from build123d import *

# Parameters (mm, degrees)
CROQUIS2_R               = 2.5
SALIENTE_EXTRUIR1_DEPTH  = 8
CROQUIS3_R               = 3.5
CORTAR_EXTRUIR1_DEPTH    = 1
CORTAR_EXTRUIR2_START    = -1
CROQUIS4_R               = 3.5
CORTAR_EXTRUIR2_DEPTH    = 1
BOSS_EXTRUDE1_DEPTH      = 10
BOSS_EXTRUDE1_DEPTH_BACK = 18
CUT_EXTRUDE1_DEPTH       = 10
CUT_EXTRUDE2_DEPTH       = 46
CUT_EXTRUDE2_DEPTH_BACK  = 31


with BuildPart() as part:
    # Croquis2 → Saliente-Extruir1 (new body)
    with BuildSketch(Plane(origin=(0, 0, 0), x_dir=(1, 0, 0), z_dir=(0, 1, 0))):
        with BuildLine():
            Line((-6.5, 70), (-6.5, 0))
            ThreePointArc((-6.5, 0), (0, -6.5), (6.5, 0))
            Line((6.5, 0), (6.5, 24))
            ThreePointArc((6.5, 24), (9.428932188, 31.071067812), (16.5, 34))
            Line((16.5, 34), (19.5, 34))
            Line((19.5, 34), (21.621320344, 36.121320344))
            Line((21.621320344, 36.121320344), (19.621320344, 38.121320344))
            Line((19.621320344, 38.121320344), (21.621320344, 40.121320344))
            Line((21.621320344, 40.121320344), (19.621320344, 42.121320344))
            Line((19.621320344, 42.121320344), (21.621320344, 44.121320344))
            ThreePointArc((21.621320344, 44.121320344), (15.831267135, 61.441250358), (13.535653981, 79.558503244))
            Line((13.535653981, 79.558503244), (11.21874212, 81.180822395))
            Line((11.21874212, 81.180822395), (12.841061271, 83.497734256))
            Line((12.841061271, 83.497734256), (10.524149409, 85.120053407))
            Line((10.524149409, 85.120053407), (12.14646856, 87.436965268))
            Line((12.14646856, 87.436965268), (9.829556699, 89.059284419))
            Line((9.829556699, 89.059284419), (11.451875849, 91.37619628))
            Line((11.451875849, 91.37619628), (11.174038765, 92.951888685))
            Line((11.174038765, 92.951888685), (6.25, 92.083647797))
            Line((6.25, 92.083647797), (-6.5, 70))
        make_face()
        with Locations(Location((0, 0, 0), (0, 0, 270))):
            Circle(CROQUIS2_R, mode=Mode.SUBTRACT)
        with Locations(Location((0, 30, 0), (0, 0, 270))):
            Circle(CROQUIS2_R, mode=Mode.SUBTRACT)
    extrude(amount=SALIENTE_EXTRUIR1_DEPTH)

    # Croquis3 → Cortar-Extruir1 (cut)
    # profile 1 of 3: a face of its own
    with BuildSketch(Plane(origin=(0, 8, 0), x_dir=(1, 0, 0), z_dir=(0, 1, 0))):
        with BuildLine():
            Line((7.515743149, 90.275979241), (-4.460249568, 69.532951382))
            Line((-4.460249568, 69.532951382), (14.458313138, 58.610314111))
            ThreePointArc((14.458313138, 58.610314111), (13.59841994, 62.277167356), (12.884475402, 65.975209032))
            Line((12.884475402, 65.975209032), (8.566911861, 90.461328646))
            Line((8.566911861, 90.461328646), (7.515743149, 90.275979241))
        make_face()
    # profile 2 of 3: a face of its own
    with BuildSketch(Plane(origin=(0, 8, 0), x_dir=(1, 0, 0), z_dir=(0, 1, 0))):
        with BuildLine():
            Line((-4.5, 67.246500228), (-4.5, 43.866114746))
            Line((-4.5, 43.866114746), (18.28754604, 43.866114746))
            Line((18.28754604, 43.866114746), (18.28754604, 46.866114746))
            ThreePointArc((18.28754604, 46.866114746), (16.631849149, 51.330235949), (15.201783832, 55.871670029))
            Line((15.201783832, 55.871670029), (-4.5, 67.246500228))
        make_face()
    # profile 3 of 3: a face of its own
    with BuildSketch(Plane(origin=(0, 8, 0), x_dir=(1, 0, 0), z_dir=(0, 1, 0))):
        with BuildLine():
            Line((-4.5, 2.828427125), (-4.5, 41.866114746))
            Line((-4.5, 41.866114746), (18.28754604, 41.866114746))
            Line((18.28754604, 41.866114746), (18.28754604, 35.866114746))
            ThreePointArc((18.28754604, 35.866114746), (8.672182695, 33.095343657), (4.5, 24))
            Line((4.5, 24), (4.5, 2.828427125))
            Line((4.5, 2.828427125), (3.5, 2.828427125))
            ThreePointArc((3.5, 2.828427125), (0, 4.5), (-3.5, 2.828427125))
            Line((-3.5, 2.828427125), (-4.5, 2.828427125))
        make_face()
        with Locations(Location((0, 30, 0), (0, 0, 270))):
            Circle(CROQUIS3_R, mode=Mode.SUBTRACT)
    extrude(amount=-CORTAR_EXTRUIR1_DEPTH, mode=Mode.SUBTRACT)

    # Croquis4 → Cortar-Extruir2 (cut)
    # profile 1 of 3: a face of its own
    with BuildSketch(Plane.XZ.offset(CORTAR_EXTRUIR2_START)):
        with BuildLine():
            Line((4.5, -24), (4.5, -2.828427125))
            Line((4.5, -2.828427125), (3.5, -2.828427125))
            ThreePointArc((3.5, -2.828427125), (0, -4.5), (-3.5, -2.828427125))
            Line((-3.5, -2.828427125), (-4.5, -2.828427125))
            Line((-4.5, -2.828427125), (-4.5, -41.866114746))
            Line((-4.5, -41.866114746), (18.28754604, -41.866114746))
            Line((18.28754604, -41.866114746), (18.28754604, -35.866114746))
            ThreePointArc((18.28754604, -35.866114746), (8.672182695, -33.095343657), (4.5, -24))
        make_face()
        with Locations(Location((0, -30, 0), (0, 0, 90))):
            Circle(CROQUIS4_R, mode=Mode.SUBTRACT)
    # profile 2 of 3: a face of its own
    with BuildSketch(Plane.XZ.offset(CORTAR_EXTRUIR2_START)):
        with BuildLine():
            Line((14.458313138, -58.610314111), (-4.460249568, -69.532951382))
            Line((-4.460249568, -69.532951382), (7.515743149, -90.275979241))
            Line((7.515743149, -90.275979241), (8.566911861, -90.461328646))
            Line((8.566911861, -90.461328646), (12.884475402, -65.975209032))
            ThreePointArc((12.884475402, -65.975209032), (13.59841994, -62.277167356), (14.458313138, -58.610314111))
        make_face()
    # profile 3 of 3: a face of its own
    with BuildSketch(Plane.XZ.offset(CORTAR_EXTRUIR2_START)):
        with BuildLine():
            Line((-4.5, -67.246500228), (15.201783832, -55.871670029))
            ThreePointArc((15.201783832, -55.871670029), (16.631849149, -51.330235949), (18.28754604, -46.866114746))
            Line((18.28754604, -46.866114746), (18.28754604, -43.866114746))
            Line((18.28754604, -43.866114746), (-4.5, -43.866114746))
            Line((-4.5, -43.866114746), (-4.5, -67.246500228))
        make_face()
    extrude(amount=CORTAR_EXTRUIR2_DEPTH, mode=Mode.SUBTRACT)

    # Sketch1 → Boss-Extrude1 (add, two sides: drawn at the far end of the back side and taken through both)
    with BuildSketch(Plane(origin=(0, 0, 0), x_dir=(-1, 0, 0), z_dir=(0, -1, 0)).offset(-BOSS_EXTRUDE1_DEPTH_BACK)):
        Polygon((-10.725693632, 78.218268839), (-13.535653981, 79.558503244), (-11.21874212, 81.180822395), (-12.841061271, 83.497734256), (-10.524149409, 85.120053407), (-12.14646856, 87.436965268), (-9.829556699, 89.059284419), (-11.451875849, 91.37619628), (-11.174038765, 92.951888685), (-8.712019383, 92.517768241), align=None)
    extrude(amount=BOSS_EXTRUDE1_DEPTH + BOSS_EXTRUDE1_DEPTH_BACK)

    # Sketch2 → Cut-Extrude1 (cut)
    with BuildSketch(Plane.XZ):
        Polygon((20.854717439, -45.882271987), (20.061595797, -46.675393628), (20.061595797, -47.817063384), (19.020844567, -48.857814614), (19.213403829, -50.036558505), (18.345213154, -50.90474918), (18.63507803, -51.655887227), (18.345213154, -51.655887227), (18.345213154, -52.50502864), (17.475337304, -52.840714546), (17.942236404, -53.732571601), (17.475337304, -53.732571601), (17.731860677, -54.397310522), (17.060300562, -55.068870638), (17.333638858, -55.705905614), (17.060300562, -55.705905614), (17.060300562, -56.646563198), (16.631849149, -57.159208559), (16.631849149, -58.201545628), (15.831267135, -59.159448073), (16.233608031, -59.750840851), (15.363432322, -60.342845501), (15.831267135, -61.441250358), (15.015003687, -61.996577004), (15.474048684, -63.074344715), (14.594646883, -63.672626132), (15.180653556, -64.533985534), (14.340267552, -65.105723423), (14.855378114, -66.315124537), (13.915417538, -66.954605767), (14.589004763, -67.944698058), (13.915417538, -68.402958115), (14.367306345, -69.46392418), (13.490959077, -70.060127513), (14.163271241, -71.048345618), (13.268305135, -72.119179344), (13.978614858, -72.712831852), (13.268305135, -73.562722816), (13.824014096, -74.379548221), (13.268305135, -74.757612427), (13.740518299, -75.451709043), (12.802233755, -76.090050022), (13.62576872, -77.300547474), (12.802233755, -77.860821134), (13.553992685, -78.96581644), align=None)
    extrude(amount=-CUT_EXTRUDE1_DEPTH, mode=Mode.SUBTRACT)

    # Sketch3 → Cut-Extrude2 (cut, two sides: drawn at the far end of the back side and taken through both)
    with BuildSketch(Plane(origin=(0, 1, 0), x_dir=(-1, 0, 0), z_dir=(0, -1, 0)).offset(-CUT_EXTRUDE2_DEPTH_BACK)):
        Polygon((-19.61873043, 25.285830451), (-7.041341817, 97.124082603), (-21.40830892, 99.639440689), (-35.796516216, 28.118225347), align=None)
    extrude(amount=CUT_EXTRUDE2_DEPTH + CUT_EXTRUDE2_DEPTH_BACK, mode=Mode.SUBTRACT)


solid = part.part
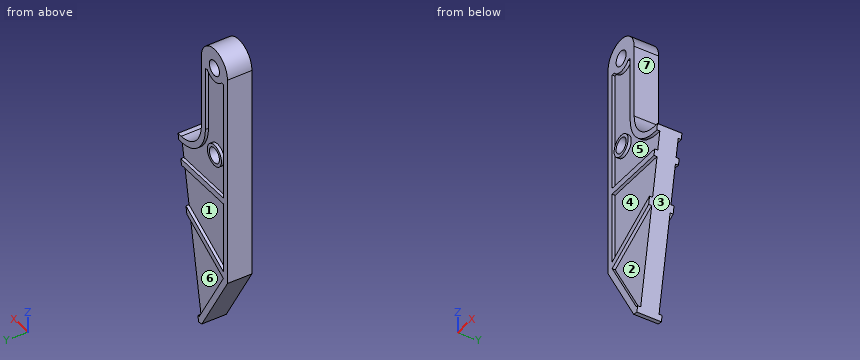
CAD build for the part. Positions are in the model's coordinates, mm. Face numbers are marked on the shaded views. A direction names the side the tool comes from. Give positions to 0.01 mm unless a question says otherwise; leave off trailing zeros. Write each loop counter-clockwise with the first axis right and the second up, starting at its lowest first coordinate (ties: lowest second). Pieces come first, ordered by that corner, then holes. Notation, with made-up numbers: (22, -22) - (63, -22) arc R20 cw to (63, -6) - close; hole circle Ø1 at (44.5, 52.25). An arc over 180 degrees is marked (long way). Answer as CSV lines item,"result".
Q1. Pull direction X, two halves, no side cores. Call the marked faces 5, 6 and 7: released by +X, released by -X, zero draft, split by the parting line, or undercut.
Result set:
face 5,"undercut"
face 6,"zero draft"
face 7,"released by +X"
Q2. Band-saw the part on C-C (x = 1). State how many separate pieces and enclosed holes the cut face has, and give its area (3 significant figures).
Result set:
separate pieces,"3"
enclosed holes,"0"
area,"515 mm²"
Q3. Band-saw the part on A-A (y = 2.75). Give the cut face in (x, z).
Result set:
outline,"(-6.5, -70) - (6.25, -92.08) - (7.87, -92.37) - (18.09, -34) - (16.5, -34) arc R10 cw to (6.5, -24) - (6.5, 0) arc R6.5 ccw to (-6.5, 0) - close; hole circle Ø5 at (0, -30); hole circle Ø5 at (0, 0)"
Q4. Flat gauge pins, fed straight in: pin 1 Ø1.5 at (x, y) = (8, 2.5) entering from +Z; pin 2 Ø0.8 at (y, z) = (0.5, -52) entering from +X; pin 3 Ø3 at (x, z) = (13.5, -67.5) entering from -Y; pin 4 Ø8 at (x, z) = (0, -30) entering from +Y. Where does each tip first touch, or does it go through?
Result set:
pin 1,"z = -27.8"
pin 2,"x = -4.5"
pin 3,"y = 1"
pin 4,"y = 8"
Q5. Drill centre lines: line 1 (Z direction, x = 0.75, y = 6.25); line 2 (Z direction, x = 12.5, y = 0.75); line 3 (Y direction, x = -0.75, z = -48). Where is each one in solid material? Low to high. Write a range as from..to.
Result set:
line 1,"-82.56..-32.38, -27.62..-2.38, 2.38..6.46"
line 2,"-59.74..-57.43, -43.87..-41.87, -35.31..-33.17"
line 3,"1..7"
Q6. 3-axis set-ups, long thin cutter, end or side, ignore diameter. For the marked faces 1, 2, 3 and 4: which of +Z, -Z, +X, -X, +Y, -Y reach the whole face in a straight line?
Result set:
face 1,"+Y"
face 2,"+X, -Y"
face 3,"-Z, +X, +Y, -Y"
face 4,"-Y"
Q7. Band-saw the part on D-D (z = -31.5). Give the cut face in (x, y).
Result set:
outline,"(-6.5, 0) - (-4.5, 0) - (-4.5, 1) - (-3.16, 1) - (-3.16, 0) - (-2, 0) - (-2, 8) - (-3.16, 8) - (-3.16, 7) - (-4.5, 7) - (-4.5, 8) - (-6.5, 8) - close; (2, 0) - (3.16, 0) - (3.16, 1) - (7.13, 1) - (7.13, 0) - (9.89, 0) - (9.89, 8) - (7.13, 8) - (7.13, 7) - (3.16, 7) - (3.16, 8) - (2, 8) - close"
Q8. Band-saw the part on B-B (z = -1). Give the cut face in (x, y), and give its area (3 significant figures).
Result set:
outline,"(-6.5, 0) - (-2.29, 0) - (-2.29, 8) - (-6.5, 8) - close; (2.29, 0) - (6.5, 0) - (6.5, 8) - (2.29, 8) - close"
area,"67.3 mm²"
